from build123d import *

# Parameters (mm, degrees)
SKETCH1_W                  = 35
SKETCH1_H                  = 45
SKETCH1_R                  = 1.5
SKETCH1_R_2                = 5
BOSS_EXTRUDE1_DEPTH        = 0.79375
CONVERT_SOLID2_START       = -0.79375
CONVERT_SOLID2_OUTLINE_W   = 35
CONVERT_SOLID2_OUTLINE_H   = 45
CONVERT_SOLID2_OUTLINE_R   = 1.5
CONVERT_SOLID2_OUTLINE_R_2 = 5
CONVERT_SOLID2_DEPTH       = 0.79375
EDGE_FLANGE1_DEPTH         = 35
EDGE_FLANGE2_DEPTH         = 35
SKETCH24_R                 = 12.4
CUT_EXTRUDE1_DEPTH         = 10
SKETCH29_W                 = 15
SKETCH29_H                 = 33.73
TAB1_DEPTH                 = 1.5875
SKETCH32_W                 = 15
SKETCH32_H                 = 33.73
TAB2_DEPTH                 = 1.5875
SKETCH35_R                 = 2.2225
CUT_EXTRUDE2_DEPTH         = 10


# Read off the part's stored shape, not the designer's step: Convert-Solid2
# Sheet-metal steps are written as plain solids
with BuildPart() as part:
    # Sketch1 → Boss-Extrude1 (new body)
    with BuildSketch(Plane.XY):
        Rectangle(SKETCH1_W, SKETCH1_H)
        with Locations((-8.5, 0)):
            Circle(SKETCH1_R, mode=Mode.SUBTRACT)
        with Locations((8.5, 0)):
            Circle(SKETCH1_R, mode=Mode.SUBTRACT)
        Circle(SKETCH1_R_2, mode=Mode.SUBTRACT)
    extrude(amount=BOSS_EXTRUDE1_DEPTH)

    # Convert-Solid2 outline → Convert-Solid2 (add)
    with BuildSketch(Plane.XY.offset(CONVERT_SOLID2_START)):
        Rectangle(CONVERT_SOLID2_OUTLINE_W, CONVERT_SOLID2_OUTLINE_H)
        with Locations((-8.5, 0)):
            Circle(CONVERT_SOLID2_OUTLINE_R, mode=Mode.SUBTRACT)
        Circle(CONVERT_SOLID2_OUTLINE_R_2, mode=Mode.SUBTRACT)
        with Locations((8.5, 0)):
            Circle(CONVERT_SOLID2_OUTLINE_R, mode=Mode.SUBTRACT)
    extrude(amount=CONVERT_SOLID2_DEPTH)

    # Edge-Flange1 section (across the edge) → Edge-Flange1 (add)
    with BuildSketch(Plane(origin=(17.5, -23.77, -0.79375), x_dir=(0, 1, 0), z_dir=(-1, 0, 0))):
        with BuildLine():
            Line((-1.5875, 1.27), (-1.5875, 35))
            Line((-1.5875, 35), (0, 35))
            Line((0, 35), (0, 1.27))
            ThreePointArc((0, 1.27), (0.371974388, 0.371974388), (1.27, 0))
            Line((1.27, 0), (1.27, -1.5875))
            ThreePointArc((1.27, -1.5875), (-0.750557627, -0.750557627), (-1.5875, 1.27))
        make_face()
    extrude(amount=EDGE_FLANGE1_DEPTH)

    # Edge-Flange2 section (across the edge) → Edge-Flange2 (add)
    with BuildSketch(Plane(origin=(17.5, -23.77, -36.79375), x_dir=(0, 0, 1), z_dir=(-1, 0, 0))):
        with BuildLine():
            Line((-1.5875, 1), (-1.5875, 46))
            Line((-1.5875, 46), (0, 46))
            Line((0, 46), (0, 1))
            ThreePointArc((0, 1), (0.292893219, 0.292893219), (1, 0))
            Line((1, 0), (1, -1.5875))
            ThreePointArc((1, -1.5875), (-0.829638796, -0.829638796), (-1.5875, 1))
        make_face()
    extrude(amount=EDGE_FLANGE2_DEPTH)

    # Sketch24 → Cut-Extrude1 (cut)
    with BuildSketch(Plane(origin=(0, 0, -38.38125), x_dir=(-1, 0, 0), z_dir=(0, 0, -1))):
        with Locations(Location((0, 0, 0), (0, 0, 90))):
            Circle(SKETCH24_R)
    extrude(amount=-CUT_EXTRUDE1_DEPTH, mode=Mode.SUBTRACT)

    # Sketch29 → Tab1 (add)
    with BuildSketch(Plane(origin=(0, -23.77, 0), x_dir=(1, 0, 0), z_dir=(0, 1, 0))):
        with Locations((25, 18.92875)):
            Rectangle(SKETCH29_W, SKETCH29_H)
    extrude(amount=-TAB1_DEPTH)

    # Sketch32 → Tab2 (add)
    with BuildSketch(Plane(origin=(0, -23.77, 0), x_dir=(1, 0, 0), z_dir=(0, 1, 0))):
        with Locations((-25, 18.92875)):
            Rectangle(SKETCH32_W, SKETCH32_H)
    extrude(amount=-TAB2_DEPTH)

    # Sketch35 → Cut-Extrude2 (cut)
    with BuildSketch(Plane(origin=(0, -23.77, 0), x_dir=(1, 0, 0), z_dir=(0, 1, 0))):
        with Locations(Location((22.5, 7.06375, 0), (0, 0, 270))):
            Circle(SKETCH35_R)
        with Locations(Location((27.5, 30.79375, 0), (0, 0, 270))):
            Circle(SKETCH35_R)
    cut_extrude2 = extrude(amount=-CUT_EXTRUDE2_DEPTH, mode=Mode.SUBTRACT)

    # Mirror1: Cut-Extrude2 across plane
    add(cut_extrude2.mirror(Plane(origin=(0, 0, 0), x_dir=(0, 0, 1), z_dir=(1, 0, 0))), mode=Mode.SUBTRACT)


solid = part.part
Read the model definition and answer for the solid it produces. Units are mm, in the model's axes. A direction names the side the tool comes from. Coordinates: 2 decimals unless noted, no trailing zeros. Write each loop counter-clockwise with the first axis right and the second up, starting at its lowest first coordinate (ties: lowest second). Pieces come first, ordered by that corner, then holes. Notation, with made-up numbers: (-30.75, 50) -> (24.25, 50) arc R20 ccw to (24.25, 68) -> close; hole circle Ø3 at (-30, -19.75). An arc over 180 degrees is marked (long way). Return JSON: item names as keys, results as strings.
(1) The part is cut by section B-B on x = 22.5. Give the vertices of the cut face in (y, z), then the cut area to 3 significant figures.
Answers below:
{"outline": "(-25.36, -35.79) -> (-23.77, -35.79) -> (-23.77, -9.29) -> (-25.36, -9.29) -> close; (-25.36, -4.84) -> (-23.77, -4.84) -> (-23.77, -2.06) -> (-25.36, -2.06) -> close", "area": "46.5 mm^2"}
(2) The part is cut by section D-D on x = 0. Give the vertices of the cut face in (y, z) (1 decimal), then the cut area to 3 significant figures.
Answers below:
{"outline": "(-25.4, -35.8) arc R2.6 ccw to (-22.8, -38.4) -> (-12.4, -38.4) -> (-12.4, -36.8) -> (-22.8, -36.8) arc R1 cw to (-23.8, -35.8) -> (-23.8, -2.1) arc R1.3 cw to (-22.5, -0.8) -> (-5, -0.8) -> (-5, 0.8) -> (-22.5, 0.8) arc R2.9 ccw to (-25.4, -2.1) -> close; (5, -0.8) -> (22.5, -0.8) -> (22.5, 0.8) -> (5, 0.8) -> close; (12.4, -38.4) -> (22.2, -38.4) -> (22.2, -36.8) -> (12.4, -36.8) -> close", "area": "151 mm^2"}
(3) Consider line 1 along Z through (x, y) = (-11.5, -14.5); line 2 along Y through (x, z) = (2.5, -13); line 3 along Z through (x, y) = (-22.5, -24.35). Determine where each line is inside the solid, lowest interval first. Write a range as from..to.
Answers below:
{"line 1": "-38.38..-36.79, -0.79..0.79", "line 2": "-25.36..-23.77", "line 3": "-35.79..-9.29, -4.84..-2.06"}
(4) Each of these flat-tipped pins is pushed along its axis until it touches: P1, Ø2.5, axis at x = 22.5, z = -7.06, coming from the +Y side; P2, Ø0.5, axis at x = -28.5, y = -25, coming from the -Z side; P3, Ø1.5, axis at x = -0.5, y = 10, coming from the -Z side; P4, Ø5, axis at x = -24.5, z = -16, coming from the +Y side. Where does it stop, or does it pass through?
Answers below:
{"P1": "through", "P2": "z = -35.79", "P3": "z = -0.79", "P4": "y = -23.77"}
(5) Which of the six approach directions +Z, -Z, +X, -X, +Y, -Y give full straight-line access (tool end or side, diameter ignored) to faces 4 (the flat face through (0, 22.23, -38)), 5 (the flat face through (8, 10, -36.794)), 6 (the flat face through (-25, -25, -35.794))?
Answers below:
{"face 4": "-Z, +X, -X, +Y", "face 5": "+X, -X, +Y", "face 6": "-Z, -X, +Y, -Y"}
(6) For a pull along Z with two mould halves and no side action, classify faces 1 (the cylindrical face through (3.72, 11.83, -37.6)), 2 (the cylindrical face through (-24.374, -24.553, -5.869)), 3 (the flat face through (8, -11, -38.381)) as pulls with the +Z half, pulls with the -Z half, needs draft (parallel to the pull), parting line crosses it, or undercut.
Answers below:
{"face 1": "needs draft", "face 2": "undercut", "face 3": "pulls with the -Z half"}
(7) The part is cut by section A-A on y = 17.5. Give the vertices of the cut face in (x, z), then the cut area to 3 significant figures.
Answers below:
{"outline": "(-17.5, -38.38) -> (17.5, -38.38) -> (17.5, -36.79) -> (-17.5, -36.79) -> close; (-17.5, -0.79) -> (17.5, -0.79) -> (17.5, 0.79) -> (-17.5, 0.79) -> close", "area": "111 mm^2"}
(8) The part is cut by section C-C on y = 10.5. Give the vertices of the cut face in (x, z), then the cut area to 3 significant figures.
Answers below:
{"outline": "(-17.5, -38.38) -> (-6.6, -38.38) -> (-6.6, -36.79) -> (-17.5, -36.79) -> close; (-17.5, -0.79) -> (17.5, -0.79) -> (17.5, 0.79) -> (-17.5, 0.79) -> close; (6.6, -38.38) -> (17.5, -38.38) -> (17.5, -36.79) -> (6.6, -36.79) -> close", "area": "90.2 mm^2"}
